Part print with two shaded views. Sizes in mm from the minimum x, y, z corner. A direction names the side the tool comes from. Round coordinates to 2 decimals unless told otherwise and drop trailing zeros. Write each loop counter-clockwise with the first axis right and the second up, starting at its lowest first coordinate (ties: lowest second). Pieces come first, ordered by that corner, then holes. Notation, with made-up numbers: (70, 16.5) -> (115, 16.5) arc R22 cw to (115, 28.5) -> close; hole circle Ø5 at (15, -22.75). An arc over 180 degrees is marked (long way). Return JSON: item names as keys, results as strings.
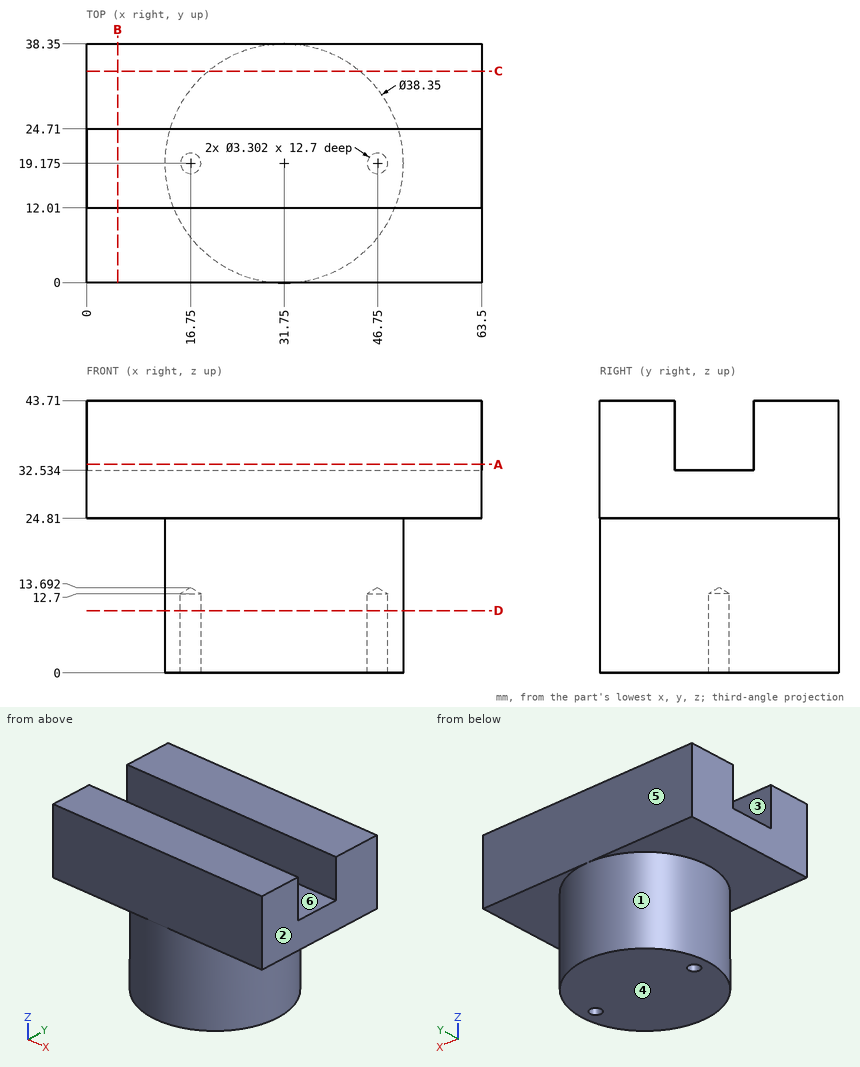
Q1. Saw through at A-A on z = 33.5. List the corners of the cut face in (x, y), then the cut area to 3 significant figures.
Verdict:
{"outline": "(0, 0) -> (63.5, 0) -> (63.5, 12.01) -> (0, 12.01) -> close; (0, 24.71) -> (63.5, 24.71) -> (63.5, 38.35) -> (0, 38.35) -> close", "area": "1,630 mm²"}
Q2. Saw through at C-C on y = 34. List the corners of the cut face in (x, z), then the cut area to 3 significant figures.
Verdict:
{"outline": "(0, 24.81) -> (19.59, 24.81) -> (19.59, 0) -> (43.91, 0) -> (43.91, 24.81) -> (63.5, 24.81) -> (63.5, 43.71) -> (0, 43.71) -> close", "area": "1,800 mm²"}
Q3. 3-axis set-ups, long thin cutter, end or side, ignore diameter. For the marked faces 1, 2 and 3: which of +Z, -Z, +X, -X, +Y, -Y reach the whole face in a straight line?
Verdict:
{"face 1": "-Z", "face 2": "+Z, -Z, +X, +Y, -Y", "face 3": "+Z, +X, -X"}
Q4. Wall check: L1, parallel to Y at x = 7, z = 41; L2, parallel to Z at x = 56, y = 13; L3, parallel to Z at x = 7.5, y = 27. Give the ranges that are in metal, low to high.
Verdict:
{"L1": "y = 0 to 12.01, 24.71 to 38.35", "L2": "z = 24.81 to 32.53", "L3": "z = 24.81 to 43.71"}
Q5. Two-plate mould, pull along Y, no slides. Class the marked faces 4, 5 and 6: +Y half, -Y half, draft (parallel to the pull), parting line (faces both ways), or undercut.
Verdict:
{"face 4": "draft", "face 5": "+Y half", "face 6": "undercut"}
Q6. Pin check, flat tips, straight feed: pin 1 Ø10 at (y, z) = (30.5, 8.5) entering from +X; pin 2 Ø8 at (x, y) = (8.5, 19.5) entering from +Z; pin 3 Ø9.5 at (x, y) = (17.5, 19) entering from -Z; pin 4 Ø2 at (x, y) = (46.75, 19.175) entering from -Z. Stop position of each tip, or through.
Verdict:
{"pin 1": "stops at x = 49.85", "pin 2": "stops at z = 32.53", "pin 3": "stops at z = 0", "pin 4": "stops at z = 13.09"}
Q7. Saw through at B-B on x = 5. List the corners of the cut face in (y, z).
Verdict:
{"outline": "(0, 24.81) -> (38.35, 24.81) -> (38.35, 43.71) -> (24.71, 43.71) -> (24.71, 32.53) -> (12.01, 32.53) -> (12.01, 43.71) -> (0, 43.71) -> close"}
Q8. Saw through at D-D on z = 10. List the corners of the cut face in (x, y) (3 decimals), then the cut area to 3 significant figures.
Verdict:
{"outline": "circle Ø38.35 at (31.75, 19.175); hole circle Ø3.302 at (16.75, 19.175); hole circle Ø3.302 at (46.75, 19.175)", "area": "1,140 mm²"}
